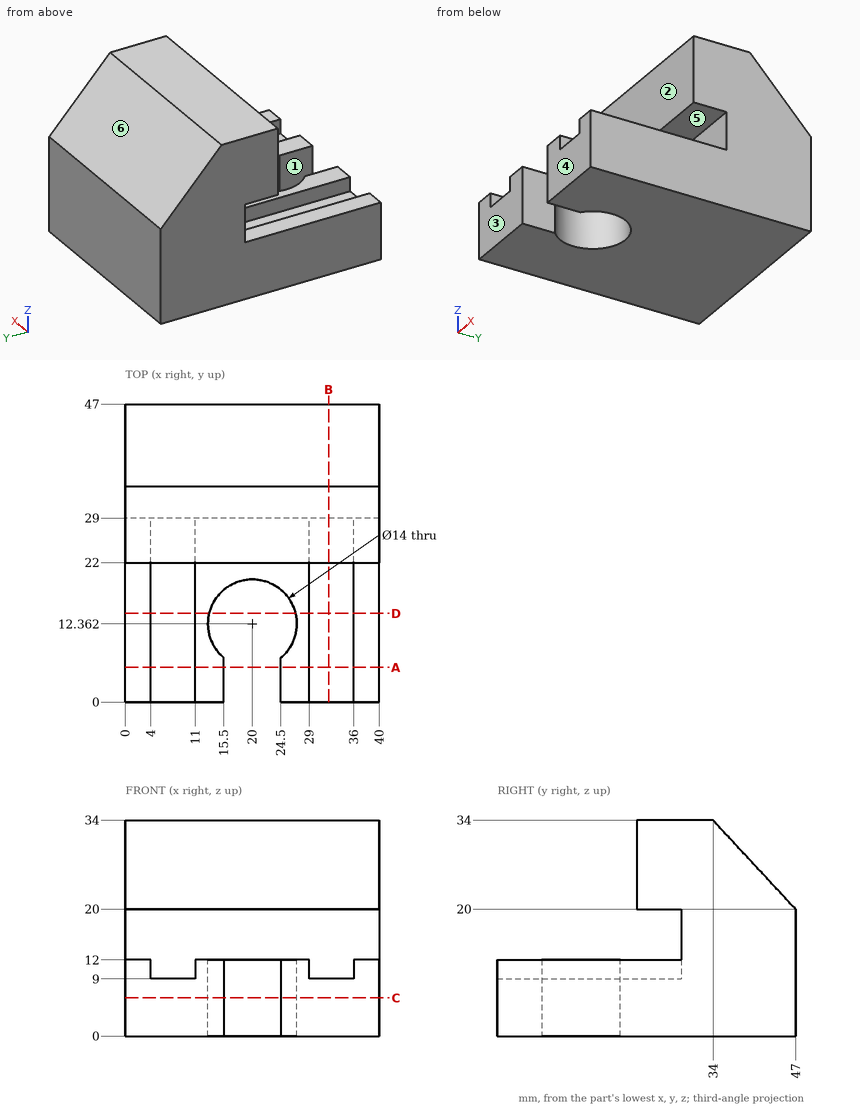
Here's the drawing with two shaded views (mm, measured from the low corner). I have some questions. A direction names the side the tool comes from. Coordinates: 2 decimals unless noted, no trailing zeros. Write each loop counter-clockwise with the first axis right and the second up, starting at its lowest first coordinate (ties: lowest second). Pieces come first, ordered by that corner, then holes. Notation, with made-up numbers: M 23.25,31 L 36.25,31 A27 ccw 36.25,70 Z; hole C -33,-8.5 d3. An arc over 180 degrees is marked long. Use one line per item in the form item = value.
Q1. For the marked faces 1, 2 and 3, which set-ups out of +Z, -Z, +X, -X, +Y, -Y let a thin tool reach every point of the face, with its end or its side?
Model answer:
face_1 = +Z, -Z, -Y
face_2 = +Z, +X, -X, -Y
face_3 = +Z, -Z, +X, -X, -Y
Q2. If we section it at D-D (y = 14): Write out the boundary of the cut face in (x, z).
Model answer:
outline = M 0,0 L 13.19,0 L 13.19,12 L 11,12 L 11,9 L 4,9 L 4,12 L 0,12 Z; M 26.81,0 L 40,0 L 40,12 L 36,12 L 36,9 L 29,9 L 29,12 L 26.81,12 Z
Q3. If we section it at B-B (x = 32): Write out the boundary of the cut face in (y, z).
Model answer:
outline = M 0,0 L 47,0 L 47,20 L 34,34 L 22,34 L 22,20 L 29,20 L 29,9 L 0,9 Z
Q4. For P1, Ø15.5, axis at x = 24, z = 26.5, coming from the -Y side; P2, Ø3, axis at x = 38, y = 12.5, coming from the +Z side; P3, Ø3, axis at x = 9.5, z = 22.5, coming from the +Y side, each with a flat end and sliding along its axis, tell me the tip position at first contact or that it passes through.
Model answer:
P1 = 22
P2 = 12
P3 = 46.07
Q5. If we section it at A-A (y = 5.5): Write out the boundary of the cut face in (x, z).
Model answer:
outline = M 0,0 L 15.5,0 L 15.5,12 L 11,12 L 11,9 L 4,9 L 4,12 L 0,12 Z; M 24.5,0 L 40,0 L 40,12 L 36,12 L 36,9 L 29,9 L 29,12 L 24.5,12 Z
Q6. If we section it at C-C (z = 6): Write out the boundary of the cut face in (x, y), then the cut area to 3 significant figures.
Model answer:
outline = M 0,0 L 15.5,0 L 15.5,7 A7 cw long 24.5,7 L 24.5,0 L 40,0 L 40,47 L 0,47 Z
area = 1,670 mm^2
Q7. We'd pull the mould along Z, two halves only. Please class the marked faces 4, 5 and 6: +Z half, -Z half, draft (parallel to the pull), parting line (faces both ways), or undercut.
Model answer:
face_4 = draft
face_5 = undercut
face_6 = +Z half
Q8. I need wall thicknesses on line 1 along Z through (x, y) = (21.5, 25.5); line 2 along Y through (x, z) = (17.5, 16.5); line 3 along Z through (x, y) = (27, 10). Which ranges of each line are inside material? Lowest first, please. Write a range as from..to.
Model answer:
line_1 = 0..12, 20..34
line_2 = 29..47
line_3 = 0..12
